Work out the finished part from the listing and answer in its coordinate system (mm). A direction names the side the tool comes from. Coordinates: 2 decimals unless noted, no trailing zeros. Order: outer loops, then holes, each group sorted by start corner. A loop starts at its lowest first (then second) coordinate and runs counter-clockwise, first axis right, second up. Notation, with made-up numbers: (61.5, 84) -> (120.5, 84) arc R21 ccw to (120.5, 89) -> close; hole circle Ø5 at (53, 16). An arc over 180 degrees is marked (long way). Write item = value, one per line. Start each with the question number.
Q1. The part is cut by section B-B, the plane x = 35. Determine the outline of the cut face in (y, z), plus the area to 3 significant figures.
Q2. Flat-ended cylindrical pins translate along their axes: pin 1 (1.5 mm diameter, centred on y = 4, z = 13, fed in from -X); pin 2 (2.5 mm diameter, centred on x = 39, z = -53.86, fed in from -Y); pin 3 (4 mm diameter, centred on x = -39, z = -53.86, fed in from +Y); pin 4 (3 mm diameter, centred on x = 7.5, y = 4.5, fed in from -Z). Find the tip coordinate at first contact, or state that the pin passes through.
Q3. Straight lines are drawn through the part: L1, parallel to X at y = 4.75, z = 48.5; L2, parallel to Y at x = 32, z = 18.5; L3, parallel to Z at x = 6, y = 2.75. For each, find the intervals that lie inside material, in ascending order. Write a range as from..to.
Q4. The part is cut by section C-C, the plane y = 4.25. Determine the outline of the cut face in (x, z), plus the area to 3 significant figures.
Q5. Which of the six approach directions +Z, -Z, +X, -X, +Y, -Y give full straight-line access (tool end or side, diameter ignored) to faces 1 (the flat face through (-40.5, 3, 11)), 2 (the flat face through (-2, 3, 70.137)), 3 (the flat face through (37.5, 3, 11)), 4 (the flat face through (-2, 3, -48.863))?
Q6. The part is cut by section D-D, the plane z = 19. Determine the outline of the cut face in (x, y).
Q7. The part is cut by section A-A, the plane z = 67.5. Determine the outline of the cut face in (x, y), plus the area to 3 significant figures.
```python
from build123d import *

# Parameters (mm, degrees)
SKETCH1_W           = 78
SKETCH1_H           = 119
BOSS_EXTRUDE1_DEPTH = 6
SKETCH1_3_R         = 1.5
SKETCH1_3_W         = 78
SKETCH1_3_H         = 119
BOSS_EXTRUDE2_DEPTH = 1
SKETCH2_W           = 66
SKETCH2_H           = 110
BOSS_EXTRUDE3_DEPTH = 0.1


with BuildPart() as part:
    # Sketch1 → Boss-Extrude1 (new body)
    with BuildSketch(Plane(origin=(0, 0, 0), x_dir=(1, 0, 0), z_dir=(0, 1, 0))):
        with Locations((-1.5, -10.636986301)):
            Rectangle(SKETCH1_W, SKETCH1_H)
    extrude(amount=BOSS_EXTRUDE1_DEPTH)

    # Sketch1_3 → Boss-Extrude2 (add)
    with BuildSketch(Plane(origin=(0, 0, 0), x_dir=(1, 0, 0), z_dir=(0, 1, 0))):
        with BuildLine():
            Line((-39, 56.863013699), (39, 56.863013699))
            ThreePointArc((39, 56.863013699), (41.121320344, 55.984334042), (42, 53.863013699))
            Line((42, 53.863013699), (42, -74.136986301))
            ThreePointArc((42, -74.136986301), (41.121320344, -76.258306645), (39, -77.136986301))
            Line((39, -77.136986301), (-39, -77.136986301))
            ThreePointArc((-39, -77.136986301), (-41.121320344, -76.258306645), (-42, -74.136986301))
            Line((-42, -74.136986301), (-42, 53.863013699))
            ThreePointArc((-42, 53.863013699), (-41.121320344, 55.984334042), (-39, 56.863013699))
        make_face()
        with Locations(Location((-39, 53.863013699, 0), (0, 0, 270))):
            Circle(SKETCH1_3_R, mode=Mode.SUBTRACT)
        with Locations(Location((39, 53.863013699, 0), (0, 0, 270))):
            Circle(SKETCH1_3_R, mode=Mode.SUBTRACT)
        with Locations(Location((-39, -74.136986301, 0), (0, 0, 270))):
            Circle(SKETCH1_3_R, mode=Mode.SUBTRACT)
        with Locations(Location((39, -74.136986301, 0), (0, 0, 270))):
            Circle(SKETCH1_3_R, mode=Mode.SUBTRACT)
        with Locations((-1.5, -10.636986301)):
            Rectangle(SKETCH1_3_W, SKETCH1_3_H, mode=Mode.SUBTRACT)
    extrude(amount=BOSS_EXTRUDE2_DEPTH)

    # Sketch2 → Boss-Extrude3 (add)
    with BuildSketch(Plane(origin=(0, 6, 0), x_dir=(1, 0, 0), z_dir=(0, 1, 0))):
        with Locations((-3, -9.136986301)):
            Rectangle(SKETCH2_W, SKETCH2_H)
    extrude(amount=BOSS_EXTRUDE3_DEPTH)


solid = part.part
```
Model answer:
q1.outline = (0, -56.86) -> (1, -56.86) -> (1, -48.86) -> (6, -48.86) -> (6, 70.14) -> (1, 70.14) -> (1, 77.14) -> (0, 77.14) -> close
q1.area = 729 mm2
q2.pin_1 = -40.5
q2.pin_2 = through
q2.pin_3 = 1
q2.pin_4 = -48.86
q3.L1 = -40.5..37.5
q3.L2 = 0..6
q3.L3 = -48.86..70.14
q4.outline = (-40.5, -48.86) -> (37.5, -48.86) -> (37.5, 70.14) -> (-40.5, 70.14) -> close
q4.area = 9,280 mm2
q5.face_1 = +Z, -Z, -X, +Y
q5.face_2 = +Z, +X, -X, +Y
q5.face_3 = +Z, -Z, +X, +Y
q5.face_4 = -Z, +X, -X, +Y
q6.outline = (-42, 0) -> (42, 0) -> (42, 1) -> (37.5, 1) -> (37.5, 6) -> (30, 6) -> (30, 6.1) -> (-36, 6.1) -> (-36, 6) -> (-40.5, 6) -> (-40.5, 1) -> (-42, 1) -> close
q7.outline = (-42, 0) -> (42, 0) -> (42, 1) -> (37.5, 1) -> (37.5, 6) -> (-40.5, 6) -> (-40.5, 1) -> (-42, 1) -> close
q7.area = 474 mm2
